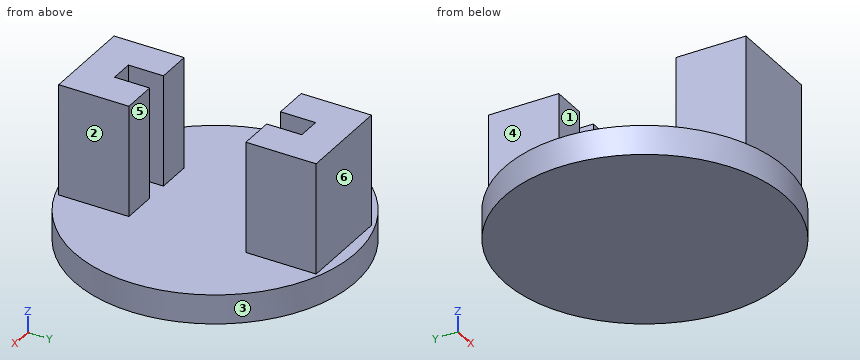
```python
from build123d import *

# Parameters (mm, degrees)
CYLINDER_R     = 12
CYLINDER_DEPTH = 2.5
BOX002_W       = 10
BOX002_H       = 10
BOX002_DEPTH   = 10
BOX001_W       = 2
BOX001_H       = 16
BOX001_DEPTH   = 10
BOX_W          = 8
BOX_H          = 22
BOX_DEPTH      = 10


with BuildPart() as cylinder:
    # Cylinder → Cylinder (new body)
    with BuildSketch(Plane.XY):
        Circle(CYLINDER_R)
    extrude(amount=CYLINDER_DEPTH)


with BuildPart() as cube002:
    # Box002 → Box002 (new body)
    with BuildSketch(Plane(origin=(-5, -5, 2), x_dir=(1, 0, 0), z_dir=(0, 0, 1))):
        with Locations((5, 5)):
            Rectangle(BOX002_W, BOX002_H)
    extrude(amount=BOX002_DEPTH)


with BuildPart() as fusion:
    # Box001 → Box001 (new body)
    with BuildSketch(Plane(origin=(-1, -8, 2), x_dir=(1, 0, 0), z_dir=(0, 0, 1))):
        with Locations((1, 8)):
            Rectangle(BOX001_W, BOX001_H)
    extrude(amount=BOX001_DEPTH)

    # Fusion: union Cube002
    add(cube002.part)


with BuildPart() as fusion001:
    # Box → Box (new body)
    with BuildSketch(Plane(origin=(-4, -11, 2), x_dir=(1, 0, 0), z_dir=(0, 0, 1))):
        with Locations((4, 11)):
            Rectangle(BOX_W, BOX_H)
    extrude(amount=BOX_DEPTH)

    # Cut: cut Fusion
    add(fusion.part, mode=Mode.SUBTRACT)

    # Fusion001: union Cylinder
    add(cylinder.part)


solid = fusion001.part
```
Could you check a few things on this model? Use its own coordinates, in mm. Face numbers are marked on the shaded views. A direction names the side the tool comes from. Coordinates: 2 decimals unless noted, no trailing zeros. Write each loop counter-clockwise with the first axis right and the second up, starting at its lowest first coordinate (ties: lowest second). Pieces come first, ordered by that corner, then holes. Notation, with made-up numbers: (-15, 39) -> (19, 39) arc R12 cw to (19, 54) -> close; hole circle Ø8 at (65.25, 62.25). An arc over 180 degrees is marked (long way). Return JSON: item names as keys, results as strings.
(1) Which directions (+Z, -Z, +X, -X, +Y, -Y) give clear straight access to the entire face, cutting with the end or side of a thin tool? Please do the marked faces 4, 5 and 6.
Numbers:
{"face 4": "+Z, -X, +Y, -Y", "face 5": "+Z, +X, -X", "face 6": "+Z, +X, -X, +Y"}
(2) We'd pull the mould along Y, two halves only. Please class the marked faces 1, 2 and 3: +Y half, -Y half, draft (parallel to the pull), parting line (faces both ways), or undercut.
Numbers:
{"face 1": "undercut", "face 2": "draft", "face 3": "parting line"}
(3) I need wall thicknesses on L1, parallel to X at y = 7.5, z = 11; L2, parallel to X at y = 9.25, z = 5.5; L3, parallel to Z at x = -8, y = -7.75. Which ranges of each line are inside material? Lowest first, please.
Numbers:
{"L1": "x = -4 to -1, 1 to 4", "L2": "x = -4 to 4", "L3": "z = 0 to 2.5"}
(4) Imagine slicing it at C-C, the plane y = 0. Please give me the cut outline in (x, z).
Numbers:
{"outline": "(-12, 0) -> (12, 0) -> (12, 2.5) -> (-12, 2.5) -> close"}
(5) Imagine slicing it at A-A, the plane z = 4.25. Please give me the cut outline in (x, y).
Numbers:
{"outline": "(-4, -11) -> (4, -11) -> (4, -5) -> (1, -5) -> (1, -8) -> (-1, -8) -> (-1, -5) -> (-4, -5) -> close; (-4, 5) -> (-1, 5) -> (-1, 8) -> (1, 8) -> (1, 5) -> (4, 5) -> (4, 11) -> (-4, 11) -> close"}
(6) Imagine slicing it at D-D, the plane y = 9.5. Please give me the cut outline in (x, z).
Numbers:
{"outline": "(-7.33, 0) -> (7.33, 0) -> (7.33, 2.5) -> (4, 2.5) -> (4, 12) -> (-4, 12) -> (-4, 2.5) -> (-7.33, 2.5) -> close"}
(7) I'm going to push flat-ended pins straight in: pin 1 (0.9 mm diameter, centred on y = -6, z = 7.5, fed in from -X); pin 2 (4 mm diameter, centred on x = 1, z = 6.5, fed in from +Y); pin 3 (3 mm diameter, centred on y = 8.5, z = 5.5, fed in from +X). Where does each tip first touch, or does it pass through?
Numbers:
{"pin 1": "stops at x = -4", "pin 2": "stops at y = 11", "pin 3": "stops at x = 4"}
(8) Imagine slicing it at B-B, the plane x = 0. Please give me the cut outline in (y, z).
Numbers:
{"outline": "(-12, 0) -> (12, 0) -> (12, 2.5) -> (11, 2.5) -> (11, 12) -> (8, 12) -> (8, 2.5) -> (-8, 2.5) -> (-8, 12) -> (-11, 12) -> (-11, 2.5) -> (-12, 2.5) -> close"}
